Could you check a few things on this model? Use its own coordinates, in mm. A direction names the side the tool comes from. Coordinates: 2 decimals unless noted, no trailing zeros. Order: outer loops, then holes, each group sorted by start corner. A loop starts at its lowest first (then second) coordinate and runs counter-clockwise, first axis right, second up. Notation, with made-up numbers: (48.5, 77.5) -> (85.5, 77.5) arc R18 ccw to (85.5, 87.5) -> close; hole circle Ø7 at (11.25, 8.5). An arc over 180 degrees is marked (long way). Return JSON: item names as keys, results as strings. Group by question number.
from build123d import *

# Parameters (mm, degrees)
SKETCH1_W           = 9
SKETCH1_H           = 43.113686922
BOSS_EXTRUDE1_DEPTH = 3


with BuildPart() as part:
    # Sketch1 → Boss-Extrude1 (new body)
    with BuildSketch(Plane.XY):
        with BuildLine():
            Line((0, -82.457009142), (15.843156539, -82.457009142))
            ThreePointArc((15.843156539, -82.457009142), (37.4, -69.007009142), (58.956843461, -82.457009142))
            Line((58.956843461, -82.457009142), (80, -82.457009142))
            Line((80, -82.457009142), (80, 0))
            Line((80, 0), (0, 0))
            Line((0, 0), (0, -82.457009142))
        make_face()
        with Locations((43.8, -42.6)):
            Rectangle(SKETCH1_W, SKETCH1_H, mode=Mode.SUBTRACT)
    extrude(amount=-BOSS_EXTRUDE1_DEPTH)


solid = part.part
Q1. I need wall thicknesses on line 1 along X through (y, z) = (-60.5, -2.9); line 2 along X through (y, z) = (-77, -0.85); line 3 along Y through (x, z) = (39.5, -1.6). Which ranges of each line are inside material? Lowest first, please. Write a range as from..to.
Q2. I want a section at D-D on x = 49.5. Please give me the cut outline in (y, z), and give its area (3 significant figures).
Q3. We'd pull the mould along Y, two halves only. Please class faces 3 (the flat face through (48.3, -43, -1)), 4 (the flat face through (31, -41, 0)), 5 (the flat face through (8, -82.457, -1)): pulls with the +Y half, pulls with the -Y half, needs draft (parallel to the pull), parting line crosses it, or undercut.
Q4. I want a section at B-B on z = -1.4. Please give me the cut outline in (x, y), and give its area (3 significant figures).
Q5. I'm going to push a flat-ended pin straight in: pin 1 Ø0.9 at (x, z) = (42, -1.5) entering from -Y. Where does the tip first touch, or does it pass through?
Q6. I want a section at A-A on y = -31.5. Please give me the cut outline in (x, z), and give its area (3 significant figures).
Q7. I want a section at C-C on y = -72. Please give me the cut outline in (x, z).
Q8. On a 3-axis mill with a long thin cutter (end or side, diameter ignored), from which of +Z, -Z, +X, -X, +Y, -Y can I reach the whole of each face in a straight line? I mean faces 1 (the cylindrical face through (37.03, -69.01, -1.48)), 2 (the flat face through (44, -64.157, -1)). Say none if no direction works.
Response values:
{
 "1": {"line 1": "x = 0..39.3, 48.3..80", "line 2": "x = 0..19.52, 55.28..80", "line 3": "y = -69.1..-64.16, -21.04..0"},
 "2": {"outline": "(-72.28, -3) -> (0, -3) -> (0, 0) -> (-72.28, 0) -> close", "area": "217 mm²"},
 "3": {"face 3": "undercut", "face 4": "needs draft", "face 5": "pulls with the -Y half"},
 "4": {"outline": "(0, -82.46) -> (15.84, -82.46) arc R24 cw to (58.96, -82.46) -> (80, -82.46) -> (80, 0) -> (0, 0) -> close; hole (39.3, -64.16) -> (48.3, -64.16) -> (48.3, -21.04) -> (39.3, -21.04) -> close", "area": "5,790 mm²"},
 "5": {"pin 1": "stops at y = -69.54"},
 "6": {"outline": "(0, -3) -> (39.3, -3) -> (39.3, 0) -> (0, 0) -> close; (48.3, -3) -> (80, -3) -> (80, 0) -> (48.3, 0) -> close", "area": "213 mm²"},
 "7": {"outline": "(0, -3) -> (25.79, -3) -> (25.79, 0) -> (0, 0) -> close; (49.01, -3) -> (80, -3) -> (80, 0) -> (49.01, 0) -> close"},
 "8": {"face 1": "+Z, -Z, -Y", "face 2": "+Z, -Z"}
}
